Input: part model. Units: mm. Frame: model coordinates. A direction names the side the tool comes from. Give positions to 0.01 mm unless a question says otherwise; leave off trailing zeros. Loops run counter-clockwise (first coordinate to the right, second up) from the corner with the lowest first, then second, coordinate; pieces in that order, holes last. Notation, with made-up numbers: M 7.5,35.25 L 24.5,35.25 A20 ccw 24.5,73.25 Z; hole C 51.25,-24.5 d7. An arc over 180 degrees is marked long. One line per item, written item: value. Start each with the question number.
(1) Pull-direction query (Y, two-part tool) for faces 4 (the cylindrical face through (9.49, -0.07, 16.5)), 5 (the cylindrical face through (9.49, -0.07, -13.5)), 6 (the flat face through (2.7, -5, 0.3)), 7 (the flat face through (0, -4.5, 0.3)); classes: released by +Y, released by -Y, zero draft, split by the parting line, or undercut.
(2) Access query for faces 1 (the cylindrical face through (5, -4.5, 16)), 2 (the flat face through (9, 0, 0)), 3 (the flat face through (9.4, -2.2, 20)). Directions: +Z, -Z, +X, -X, +Y, -Y. A direction counts if a zero-diameter tool reaches every point of the face in a straight line with its end or side. Return the directions, or none.
(3) Pin query (flat end, axial travel): P1, Ø3, axis at y = 1.5, z = 2.5, coming from the -X side; P2, Ø1.8, axis at y = 0, z = 15, coming from the +X side; P3, Ø6, axis at x = 4.5, z = 7, coming from the +Y side. Return the tip coordinate at first contact, or that it passes through.
(4) Ray query, line 1 along Z through (x, y) = (9.45, 0); line 2 along Y through (x, z) = (9.3, -15); line 3 along X through (y, z) = (0.5, -5). Return the intervals inside material, ascending. Write a range as from..to.
(5) Section B-B on x = 5. Output: boundary loops of the cut face in (y, z).
(6) Section A-A on z = -13. Output: boundary loops of the cut face in (x, y).
(7) Section C-C on z = 15.5. Output: boundary loops of the cut face in (x, y).
(8) Section D-D on y = 0.75. Output: boundary loops of the cut face in (x, z).
Autodesk Inventor part; units mm, degrees
ref_plane "YZ Plane" through (0, 0, 0) normal (1, 0, 0) x (0, 1, 0)
ref_plane "XZ Plane" through (0, 0, 0) normal (0, 1, 0) x (-1, 0, 0)
ref_plane "XY Plane" through (0, 0, 0) normal (0, 0, 1) x (1, 0, 0)
sketch "スケッチ1" plane through (0, 0, 0) normal (1, 0, 0) x (0, 1, 0)
  line L0 (-5, -20) -> (5, -20)
  line L1 (5, -20) -> (5, 20)
  line L2 (5, 20) -> (-5, 20)
  line L3 (-5, 20) -> (-5, -20)
  line L4 (-5, -20) -> (5, 20) construction
  line L5 (5, -20) -> (-5, 20) construction
  point P0 (0, 0)
  dimension "d0" = 10
  dimension "d1" = 40
extrude "押し出し1" add sketch "スケッチ1" along normal blind 10
shell "シェル1" thickness 1 removed faces 4 at (3.3333, 1.6667, 20) at (3.3333, 5, -6.6667) at (3.3333, -1.6667, -20) at (0, -1.6667, 6.6667)
sketch "スケッチ2" plane through (10, 0, 0) normal (1, 0, 0) x (0, 0, -1)
  line L0 (20, -5) -> (20, 5)
  line L1 (-20, 5) -> (-20, -5)
  line L2 (20, 5) -> (-20, 5)
  point P0 (0, 0)
  point P1 (-15, 0)
  point P2 (15, 0)
  dimension "d5" = 5
  dimension "d6" = 5
  dimension "d14" = 5
hole "穴1" at (10, 0, 15) at (10, 0, -15) direction (-1, 0, 0) diameter 3 end through all
sketch "スケッチ3" plane through (0, -5, -20) normal (0, -1, 0) x (1, 0, 0)
  line L0 (7, 34) -> (7, 6)
  arc A0 (3, 6) -> (7, 6) centre (5, 6) ccw
  line L1 (3, 6) -> (3, 34)
  arc A1 (7, 34) -> (3, 34) centre (5, 34) ccw
  line L2 (0, 40) -> (10, 40)
  line L3 (0, 40) -> (0, 0)
  line L4 (0, 0) -> (10, 0)
  point P0 (0, 20)
  point P1 (3, 20)
  point P2 (0, 20)
  dimension "d15" = 2
  dimension "d17" = 5
  dimension "d22" = 6
extrude "押し出し2" cut sketch "スケッチ3" against normal blind 1
properties part number "palmrest_L_large" material "アルミニウム 6061"
Output values:
1. face 4: undercut
1. face 5: undercut
1. face 6: released by -Y
1. face 7: zero draft
2. face 1: +Y, -Y
2. face 2: +Z, -Z, -X, +Y
2. face 3: +Z, +X, -X, +Y, -Y
3. P1: stops at x = 9
3. P2: passes through
3. P3: stops at y = -4
4. line 1: z = -20..-16.5, -13.5..13.5, 16.5..20
4. line 2: y = -5..-1.5, 1.5..5
4. line 3: x = 9..10
5. outline: M -5,-20 L -4,-20 L -4,-16 L -5,-16 Z; M -5,16 L -4,16 L -4,20 L -5,20 Z
6. outline: M 0,-5 L 3,-5 L 3,-4 L 0,-4 Z; M 7,-5 L 10,-5 L 10,5 L 9,5 L 9,-4 L 7,-4 Z
7. outline: M 0,-5 L 3.68,-5 L 3.68,-4 L 0,-4 Z; M 6.32,-5 L 10,-5 L 10,-1.41 L 9,-1.41 L 9,-4 L 6.32,-4 Z; M 9,1.41 L 10,1.41 L 10,5 L 9,5 Z
8. outline: M 9,-20 L 10,-20 L 10,-16.3 L 9,-16.3 Z; M 9,-13.7 L 10,-13.7 L 10,13.7 L 9,13.7 Z; M 9,16.3 L 10,16.3 L 10,20 L 9,20 Z
